For this review, take the finished solid that the model builds, in its own axes (mm). Round coordinates to 2 decimals unless told otherwise and drop trailing zeros. Order: outer loops, then holes, each group sorted by start corner. A loop starts at its lowest first (then second) coordinate and runs counter-clockwise, first axis right, second up. Notation, with made-up numbers: (-14.5, 55.5) -> (-9.5, 55.5) arc R31 cw to (-9.5, 82.5) -> close; hole circle Ø6 at (-14, 80). An arc over 180 degrees is marked (long way). Use a Markdown table: item, result. Add a question column.
1) Consider section A-A (x = 0). State the section outline as (y, z) points.
2) Consider section D-D (z = 1.75). State the section outline as (x, y) points, plus the area to 3 significant figures.
3) Consider section B-B (y = 31). State the section outline as (x, z) points, plus the area to 3 significant figures.
4) Consider section C-C (x = 35). State the section outline as (y, z) points.
5) Clearance check with flat-ended pins moving along their axes: P1, Ø6, axis at x = -31.5, y = -11, coming from the -Z side; P2, Ø2, axis at x = -26.5, z = 3.5, coming from the +Y side; P3, Ø1.5, axis at x = 14, z = 5.5, coming from the -Y side; P4, Ø2, axis at y = -3, z = 4, coming from the +X side. State where each tip first meets the part, or that it passes through.
6) Draft analysis for pull direction Y (two halves, no side actions). For faces 1 (the face through (-3.03, 18.17, 3.45)), 2 (the face through (-14.434, -11.357, 3.451)), 3 (the face through (-38.19, -22.37, 3.45)), 4 (the face through (-6, 10, 7)), state which applies: pulls with the +Y half, pulls with the -Y half, needs draft (parallel to the pull), parting line crosses it, or undercut.
7) Wall thickness on line 1 along Y through (x, z) = (-4, 5.25); line 2 along Y through (x, z) = (0, 4.25); line 3 along X through (y, z) = (-9, 6.25): over which ranges is each line inside the solid? List them lowest first. Write a range as [from, to].
```python
from build123d import *

# Parameters (mm, degrees)
F0_R     = 10.92
F1_DEPTH = 7


# Not quite as in the source:
# - a feature names something its author has since deleted; it is built from what else it names


with BuildPart() as f1:
    # F0 (on Top) → F1 (new body)
    with BuildSketch(Plane.XY):
        with BuildLine():
            ThreePointArc((28.3529823071, 1.6761283467), (16.1276038689, 9.8932258121), (14.1316130419, 24.4876284834))
            ThreePointArc((14.1316130419, 24.4876284834), (-1.0184797386, 44.2482801815), (-15.2433325814, 23.8114940253))
            ThreePointArc((-15.2433325814, 23.8114940253), (-16.5331807129, 9.1989312159), (-28.2699008548, 0.3989255129))
            ThreePointArc((-28.2699008548, 0.3989255129), (-37.9772339165, -22.7266382845), (-12.9562617696, -24.4514481107))
            ThreePointArc((-12.9562617696, -24.4514481107), (0.5300904983, -17.9124126397), (14.291675769, -23.8503797349))
            ThreePointArc((14.291675769, -23.8503797349), (39.2470886778, -20.9610002997), (28.3529823071, 1.6761283467))
        make_face()
        with Locations((-24.849640726, -14.6369722206)):
            Circle(F0_R, mode=Mode.SUBTRACT)
        Circle(F0_R, mode=Mode.SUBTRACT)
        with Locations((25.7406966372, -13.5209886029)):
            Circle(F0_R, mode=Mode.SUBTRACT)
        with Locations((-0.6636456317, 28.8323633176)):
            Circle(F0_R, mode=Mode.SUBTRACT)
    extrude(amount=F1_DEPTH)


solid = f1.part
```
Results list:
| question | item | result |
|---|---|---|
| 1 | outline | (-17.93, 0) -> (-10.92, 0) -> (-10.92, 7) -> (-17.93, 7) -> close; (10.92, 0) -> (17.93, 0) -> (17.93, 7) -> (10.92, 7) -> close; (39.73, 0) -> (44.24, 0) -> (44.24, 7) -> (39.73, 7) -> close |
| 2 | outline | (-28.27, 0.4) arc R15.42 ccw (long way) to (-12.96, -24.45) arc R18 cw to (14.29, -23.85) arc R15.42 ccw (long way) to (28.35, 1.68) arc R18 cw to (14.13, 24.49) arc R15.42 ccw (long way) to (-15.24, 23.81) arc R18 cw to start; hole circle Ø21.84 at (-24.85, -14.64); hole circle Ø21.84 at (-0.66, 28.83); hole circle Ø21.84 at (0, 0); hole circle Ø21.84 at (25.74, -13.52) |
| 2 | area | 1,780 mm2 |
| 3 | outline | (-15.93, 0) -> (-11.37, 0) -> (-11.37, 7) -> (-15.93, 7) -> close; (10.04, 0) -> (14.6, 0) -> (14.6, 7) -> (10.04, 7) -> close |
| 3 | area | 63.9 mm2 |
| 4 | outline | (-25.85, 0) -> (-19.31, 0) -> (-19.31, 7) -> (-25.85, 7) -> close; (-7.73, 0) -> (-1.19, 0) -> (-1.19, 7) -> (-7.73, 7) -> close |
| 5 | P1 | through |
| 5 | P2 | y = 1.27 |
| 5 | P3 | y = -24.34 |
| 5 | P4 | x = 37.87 |
| 6 | face 1 | undercut |
| 6 | face 2 | undercut |
| 6 | face 3 | parting line crosses it |
| 6 | face 4 | needs draft |
| 7 | line 1 | [-18.6, -10.16], [10.16, 18.43], [39.23, 43.89] |
| 7 | line 2 | [-17.93, -10.92], [10.92, 17.93], [39.73, 44.24] |
| 7 | line 3 | [-39.2, -34.2], [-15.5, -6.18], [6.18, 15.8], [35.68, 40.48] |
